```python
from build123d import *

# Parameters (mm, degrees)
SKETCH_1_W          = 6.5
SKETCH_1_H          = 6.5
SKETCH_1_R          = 2.05
EXTRUDE_1_DEPTH     = 6.5
SKETCH_2_W          = 6.5
SKETCH_2_H          = 13
EXTRUDE_2_DEPTH     = 6.5
SKETCH_3_W          = 6.5
SKETCH_3_H          = 6.5
SKETCH_3_R          = 2.05
EXTRUDE_3_DEPTH     = 6.5
SKETCH_4_R          = 2.05
CUT_EXTRUDE_1_DEPTH = 8
FILLET_1_R          = 3
FILLET_2_R          = 3


with BuildPart() as part:
    # 草图1 → 凸台-拉伸1 (new body)
    with BuildSketch(Plane.XY):
        with Locations((-8.580694703, 4.782128964)):
            Rectangle(SKETCH_1_W, SKETCH_1_H)
        with Locations(Location((-8.580694703, 4.782128964, 0), (0, 0, 180))):
            Circle(SKETCH_1_R, mode=Mode.SUBTRACT)
    extrude(amount=EXTRUDE_1_DEPTH)

    # 草图2 → 凸台-拉伸2 (add)
    with BuildSketch(Plane(origin=(-5.330694703, 0, 0), x_dir=(0, 0, -1), z_dir=(1, 0, 0))):
        with Locations((3.25, 8.032128964)):
            Rectangle(SKETCH_2_W, SKETCH_2_H)
    extrude(amount=-EXTRUDE_2_DEPTH)

    # 草图3 → 凸台-拉伸3 (add)
    with BuildSketch(Plane(origin=(-5.330694703, 0, 0), x_dir=(0, 0, -1), z_dir=(1, 0, 0))):
        with Locations((3.25, 4.782128964)):
            Rectangle(SKETCH_3_W, SKETCH_3_H)
        with Locations(Location((3.25, 4.782128964, 0), (0, 0, 180))):
            Circle(SKETCH_3_R, mode=Mode.SUBTRACT)
    extrude(amount=EXTRUDE_3_DEPTH)

    # 草图4 → 切除-拉伸1 (cut)
    with BuildSketch(Plane(origin=(0, 14.532128964, 0), x_dir=(1, 0, 0), z_dir=(0, 1, 0))):
        with Locations(Location((-8.580694703, 3.25, 0), (0, 0, 270))):
            Circle(SKETCH_4_R)
    extrude(amount=-CUT_EXTRUDE_1_DEPTH, mode=Mode.SUBTRACT)

    # 圆角1
    fillet_1_edges = [part.edges().sort_by_distance(p)[0] for p in [
        (-5.330694703, 1.532128964, -6.5),
        (-11.830694703, 11.282128964, 0),
        (-11.830694703, 8.032128964, -6.5),
        (-5.330694703, 11.282128964, -6.5),
        (-2.080694703, 8.032128964, -6.5),
        (-11.830694703, 1.532128964, 0),
        (-11.830694703, 8.032128964, 3.25),
    ]]
    fillet(fillet_1_edges, radius=FILLET_1_R)

    # 圆角2
    # the kernel refuses this fillet: 3 mm, written as the material it adds along each edge
    with BuildSketch(Plane(origin=(-5.330694703, 1.532128964, 0), x_dir=(0, 0, 1), z_dir=(0, 1, 0))) as fillet_2_piece_1:
        with BuildLine():
            CenterArc((FILLET_2_R, FILLET_2_R), FILLET_2_R, 180, 90)
            Line((0, FILLET_2_R), (0, 0))
            Line((0, 0), (FILLET_2_R, 0))
        make_face()
    extrude(amount=6.5)


solid = part.part
```
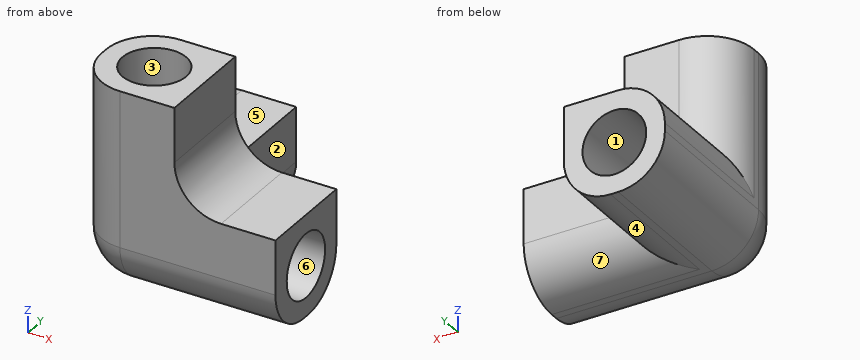
Can you work these out from the model? Positions are in its coordinate system, mm. Face numbers are marked on the shaded views. A direction names the side the tool comes from. Coordinates: 2 decimals unless noted, no trailing zeros. Order: outer loops, then holes, each group sorted by start corner. A loop starts at its lowest first (then second) coordinate and runs counter-clockwise, first axis right, second up.
1. If we section it at C-C (y = 3.5): Please give me the cut outline in (x, z), then the cut area to 3 significant figures.
2. I need wall thicknesses on line 1 (Y direction, x = -2.5, z = -3.25); line 2 (X direction, y = 12.5, z = -3.25); line 3 (X direction, y = 6.5, z = 1.5). Which ranges of each line are inside material? Lowest first, please.
3. If we section it at B-B (y = 7.75): Please give me the cut outline in (x, z).
4. Thinking about a two-plate mould opening in Y: for the marked faces 5, 6 and 7, which applies, +Y half, -Y half, draft (parallel to the pull), parting line (faces both ways), or undercut?
5. If we section it at A-A (z = -3.25): Please give me the cut outline in (x, y).
6. I'm going to push flat-ended pins straight in: pin 1 (3 mm diameter, centred on x = -8.5, y = 13, fed in from +Z); pin 2 (4 mm diameter, centred on y = 11.5, z = -1.5, fed in from +X). Where does each tip first touch, or does it pass through?
7. If we section it at D-D (x = -3.5): Please give me the cut outline in (y, z).
8. For the marked faces 1, 2, 3 and 4, which set-ups out of +Z, -Z, +X, -X, +Y, -Y let a thin tool reach every point of the face, with its end or its side?
Entries:
1. outline: (-11.65, -3.5) arc R2.82 ccw to (-8.83, -6.32) - (1.17, -6.32) - (1.17, -4.85) - (-5.33, -4.85) - (-5.33, -1.65) - (1.17, -1.65) - (1.17, 0) - (-2.33, 0) arc R3 cw to (-5.33, 3) - (-5.33, 6.5) - (-6.98, 6.5) - (-6.98, 0) - (-10.18, 0) - (-10.18, 6.5) - (-11.65, 6.5) - close
1. area: 80.7 mm2
2. line 1: y = 1.53 to 2.73, 6.83 to 8.03
2. line 2: x = -11.83 to -10.63, -6.53 to -5.33
2. line 3: x = -11.45 to -9.7, -7.46 to -4.93
3. outline: (-11.83, -3.5) arc R3 ccw to (-8.83, -6.5) - (-8.33, -6.5) arc R3 ccw to (-5.61, -4.77) - (1.17, -4.77) - (1.17, 0) - (-2.33, 0) arc R3 cw to (-5.33, 3) - (-5.33, 6.5) - (-10.1, 6.5) - (-10.1, -0.28) arc R3 ccw to (-11.83, -3) - close; hole circle Ø4.1 at (-8.58, -3.25)
4. face 5: draft
4. face 6: undercut
4. face 7: +Y half
5. outline: (-11.83, 4.53) arc R3 ccw to (-8.83, 1.53) - (1.17, 1.53) - (1.17, 2.73) - (-5.33, 2.73) - (-5.33, 6.83) - (1.17, 6.83) - (1.17, 8.03) - (-5.33, 8.03) - (-5.33, 14.53) - (-6.53, 14.53) - (-6.53, 6.53) - (-10.63, 6.53) - (-10.63, 14.53) - (-11.83, 14.53) - close
6. pin 1: stops at z = 0
6. pin 2: stops at x = -5.33
7. outline: (1.53, -3.5) arc R3 ccw to (4.53, -6.5) - (5.03, -6.5) arc R3 ccw to (8.03, -3.5) - (8.03, 0.24) - (1.53, 0.24) - close; hole circle Ø4.1 at (4.78, -3.25)
8. face 1: +Y
8. face 2: +Z, -Z, +X, +Y
8. face 3: +Z
8. face 4: -Z, +X, +Y
